CAD build for the part. Positions are in the model's coordinates, mm. Face numbers are marked on the shaded views. A direction names the side the tool comes from. Give positions to 0.01 mm unless a question says otherwise; leave off trailing zeros. Write each loop counter-clockwise with the first axis right and the second up, starting at its lowest first coordinate (ties: lowest second). Pieces come first, ordered by that corner, then holes. Notation, with made-up numbers: (-26.75, -28.5) -> (2.25, -28.5) arc R24 ccw to (2.25, 3.5) -> close; hole circle Ø2 at (64, 6.25). An arc over 180 degrees is marked (long way). Answer in a Markdown table with one row per item. Add a question column.
Autodesk Inventor part; units mm, degrees
ref_plane "YZ Plane" through (0, 0, 0) normal (1, 0, 0) x (0, 1, 0)
ref_plane "XZ Plane" through (0, 0, 0) normal (0, 1, 0) x (-1, 0, 0)
ref_plane "XY Plane" through (0, 0, 0) normal (0, 0, 1) x (1, 0, 0)
sketch "Sketch1" plane through (0, 0, 0) normal (0, 0, 1) x (1, 0, 0)
  line L0 (1.5875, 14.0208) -> (1.5875, 42.8625)
  line L1 (0, 44.45) -> (0, 14.0208)
  line L2 (6.35, 50.8) -> (31.0388, 50.8)
  line L3 (32.6263, 49.2125) -> (7.9375, 49.2125)
  arc A0 (6.35, 50.8) -> (0, 44.45) centre (6.35, 44.45) ccw
  line L4 (1.5875, 42.8625) -> (7.9375, 49.2125)
  line L5 (31.0388, 50.8) -> (31.0388, 69.85)
  line L6 (32.6263, 50.8) -> (32.6263, 69.85)
  line L7 (31.0388, 69.85) -> (32.6263, 69.85)
  line L8 (32.6263, 50.8) -> (32.6263, 49.2125)
  line L9 (0, 14.0208) -> (1.5875, 14.0208)
  point P0 (0, 0)
  point P1 (1.8599, 48.9401)
  point P2 (4.7625, 46.0375)
  dimension "d7" = 1.5875
  dimension "d8" = 19.05
  dimension "d48" = 24.6888
extrude "Extrusion1" add sketch "Sketch1" along normal blind 15.875
fillet "Fillet1" radius 1.5875 2 edges at (31.0388, 50.8, 7.9375) (32.6263, 49.2125, 7.9375)
sketch "Sketch2" plane through (32.6263, 69.85, 15.875) normal (1, 0, 0) x (0, 0, -1)
  line L0 (15.875, 0) -> (0, 0)
  point P0 (15.875, -69.85)
  point P1 (7.9375, -7.9375)
  dimension "d12" = 7.9375
sketch "Sketch5" plane through (7.9375, 49.2125, 0) normal (0, -1, 0) x (1, 0, 0)
  point P0 (-7.9375, 0)
  point P1 (8.7312, 7.9375)
sketch "Sketch6" plane through (1.5875, 14.0208, 0) normal (1, 0, 0) x (0, 0, -1)
  line L0 (0, 0) -> (-15.875, 0)
  line L1 (0, 0) -> (0, 28.8417)
  line L2 (0, 28.8417) -> (-15.875, 28.8417)
  line L3 (-15.875, 0) -> (-15.875, 28.8417)
  line L4 (0, 0) -> (-15.875, 0)
  point P0 (-7.9375, 7.9375)
  point P1 (-7.9375, 30.1625)
  dimension "d15" = 7.9375
hole "Hole2" at (16.6687, 49.2125, 7.9375) direction (0, 1, 0) diameter 4.7625 end through all countersink diameter 7.9375 countersink angle 82
hole "Hole3" at (32.6263, 61.9125, 7.9375) direction (-1, 0, 0) diameter 4.7625 end through all countersink diameter 7.9375 countersink angle 82
hole "Hole4" at (1.5875, 21.9583, 7.9375) direction (-1, 0, 0) diameter 4.7625 end through all countersink diameter 7.9375 countersink angle 82
properties part number "bracket"
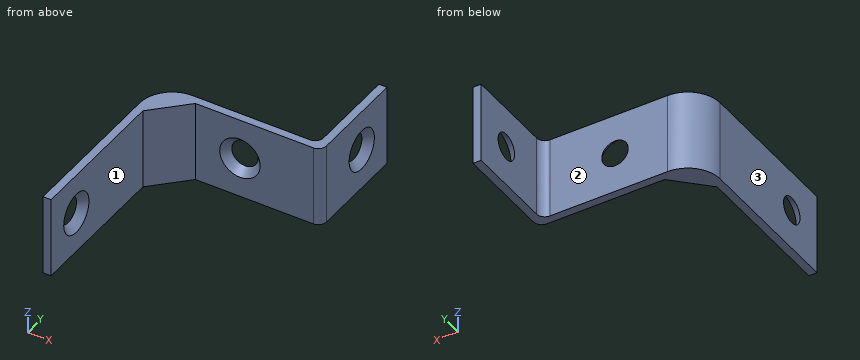
Item 1: Slice it at C-C, the plane x = 10.5. List the corners of the cut face in (y, z) (1 decimal).
Item 2: Probe L1, parallel to X at y = 30, z = 7.75; L2, parallel to Y at x = 21.5, z = 7; L3, parallel to X at y = 57.5, z = 1.5. List the from-to ranges inside material, lowest first. Write a range as from..to.
Item 3: Drop flat-ended pins along their axis: pin 1 Ø5 at (x, z) = (19.5, 11) entering from -Y; pin 2 Ø2 at (x, z) = (17.5, 3.5) entering from +Y; pin 3 Ø1.5 at (y, z) = (49, 11.5) entering from +X. Give the stop position or say it passes through.
Item 4: Which spindle directions (+Z, -Z, +X, -X, +Y, -Y) get a long thin tool onto all of the face, cutting with end or side? Do the marked faces 1, 2 and 3. Say none if no direction does.
Item 5: Slice it at D-D, the plane z = 10. State how many separate pieces and enclosed holes the cut face has, then the cut area to 3 significant figures.
Item 6: Slice it at B-B, the plane y = 29.5. List the corners of the cut face in (x, z) (1 decimal), then the cut area to 3 significant figures.
Item 7: Slice it at A-A, the plane z = 14.5. List the corners of the cut face in (x, y), then the cut area to 3 significant figures.
Answer key:
| question | item | result |
|---|---|---|
| 1 | outline | (49.2, 0) -> (50.8, 0) -> (50.8, 15.9) -> (49.2, 15.9) -> close |
| 2 | L1 | x = 0..1.59 |
| 2 | L2 | y = 49.21..50.8 |
| 2 | L3 | x = 31.04..32.63 |
| 3 | pin 1 | stops at y = 49.21 |
| 3 | pin 2 | stops at y = 50.8 |
| 3 | pin 3 | stops at x = 32.23 |
| 4 | face 1 | +Z, -Z, +X, -Y |
| 4 | face 2 | +Z, -Z, -X, +Y |
| 4 | face 3 | +Z, -Z, -X, +Y, -Y |
| 5 | separate pieces | 4 |
| 5 | enclosed holes | 0 |
| 5 | area | 125 mm² |
| 6 | outline | (0, 0) -> (1.6, 0) -> (1.6, 15.9) -> (0, 15.9) -> close |
| 6 | area | 25.2 mm² |
| 7 | outline | (0, 14.02) -> (1.59, 14.02) -> (1.59, 42.86) -> (7.94, 49.21) -> (31.04, 49.21) arc R1.59 ccw to (32.63, 50.8) -> (32.63, 69.85) -> (31.04, 69.85) -> (31.04, 52.39) arc R1.59 cw to (29.45, 50.8) -> (6.35, 50.8) arc R6.35 ccw to (0, 44.45) -> close |
| 7 | area | 149 mm² |
